```python
from build123d import *

# Parameters (mm, degrees)
SKETCH1_W           = 122
SKETCH1_H           = 105
SKETCH1_R           = 8
BOSS_EXTRUDE1_DEPTH = 3.175


with BuildPart() as part:
    # Sketch1 → Boss-Extrude1 (new body)
    with BuildSketch(Plane.XY):
        with Locations((42, -27.5)):
            Rectangle(SKETCH1_W, SKETCH1_H)
        with Locations((84.431124445, -41.275)):
            Circle(SKETCH1_R, mode=Mode.SUBTRACT)
        Circle(SKETCH1_R, mode=Mode.SUBTRACT)
    extrude(amount=-BOSS_EXTRUDE1_DEPTH)


solid = part.part
```
Geometry check sheet. Reference: the model listing, model coordinates, mm. Coordinates: 2 decimals unless noted, no trailing zeros. Write each loop counter-clockwise with the first axis right and the second up, starting at its lowest first coordinate (ties: lowest second). Pieces come first, ordered by that corner, then holes. Notation, with made-up numbers: M 72,-11 L 122,-11 A27 ccw 122,11 Z; hole C 17.25,63.5 d5. An arc over 180 degrees is marked long. One line per item, written item: value. Start each with the question number.
(1) Sectioned sample at A-A, the plane y = 0. Enter the section's corners in (x, z) (3 decimals).
(2) Sectioned sample at C-C, the plane z = -1.4. Enter the section's corners in (x, y) (3 decimals).
(3) Sectioned sample at B-B, the plane x = -2.5. Enter the section's corners in (y, z) (3 decimals), and give its area (3 significant figures).
(4) Release check for a two-part mould opening along Y. For faces 1 (the face through (41, 25, -2)), 2 (the face through (41, -27, -3.175)), 3 (the face through (-1.73, -7.81, -1.57)) record: released by +Y, released by -Y, zero draft, split by the parting line, or undercut.
(5) Depth check by flat-ended pin: pin 1 (9.5 mm diameter, centred on x = 0, y = 0, fed in from -Z); pin 2 (3 mm diameter, centred on x = 86, y = -53.5, fed in from +Z). Enter the tip coordinate at first touch or a pass-through.
(6) Scan lines: line 1 along Y through (x, z) = (0, -2.05); line 2 along Y through (x, z) = (-4.5, -2.3). Record each from-to range of solid material in increasing order. Write a range as [from, to].
Filled sheet:
1. outline: M -19,-3.175 L -8,-3.175 L -8,0 L -19,0 Z; M 8,-3.175 L 103,-3.175 L 103,0 L 8,0 Z
2. outline: M -19,-80 L 103,-80 L 103,25 L -19,25 Z; hole C 0,0 d16; hole C 84.431,-41.275 d16
3. outline: M -80,-3.175 L -7.599,-3.175 L -7.599,0 L -80,0 Z; M 7.599,-3.175 L 25,-3.175 L 25,0 L 7.599,0 Z
3. area: 285 mm²
4. face 1: released by +Y
4. face 2: zero draft
4. face 3: undercut
5. pin 1: through
5. pin 2: z = 0
6. line 1: [-80, -8], [8, 25]
6. line 2: [-80, -6.61], [6.61, 25]
